Check sheet for the modelled part. Datum: model origin and axes. Units: mm. Face numbers are marked on the shaded views. Round coordinates to 2 decimals unless told otherwise and drop trailing zeros. Write each loop counter-clockwise with the first axis right and the second up, starting at its lowest first coordinate (ties: lowest second). Pieces come first, ordered by that corner, then holes. Notation, with made-up numbers: M 53.25,64.25 L 102.25,64.25 A15 cw 102.25,88.25 Z; hole C 72.5,70.25 d11. An arc over 180 degrees is marked long. Answer in a Markdown table with one row per item.
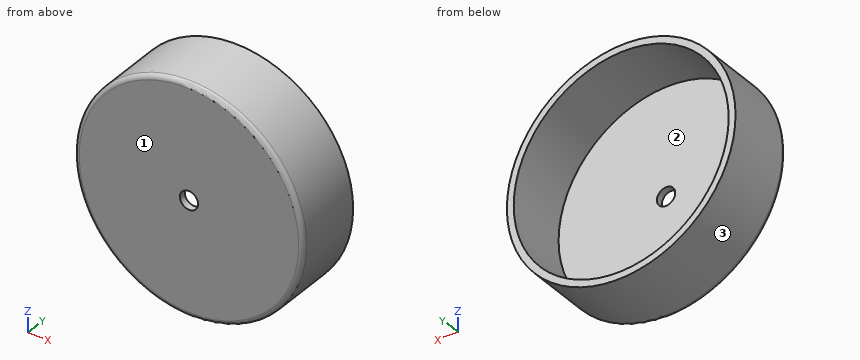
```python
from build123d import *

# Parameters (mm, degrees)
F0_R     = 50
F1_DEPTH = 30
F2_T     = -3
F3_R     = 2
F5_D     = 8


with BuildPart() as f1:
    # F0 (on Front) → F1 (new body)
    with BuildSketch(Plane.XZ):
        Circle(F0_R)
    extrude(amount=F1_DEPTH)

    # F2
    f2_openings = [f1.faces().sort_by_distance(p)[0] for p in [
        (0, 0, 0),
    ]]
    offset(amount=F2_T, openings=f2_openings)

    # F3
    f3_edges = [f1.edges().sort_by_distance(p)[0] for p in [
        (-50, -30, 0),
    ]]
    fillet(f3_edges, radius=F3_R)

    # F5 (through all)
    with Locations(Plane.XZ.offset(30)):
        with Locations((0, 0)):
            Hole(F5_D / 2)


solid = f1.part
```
1. Go/stop test with flat-tipped pins: pin 1 (1 mm diameter, centred on y = -6, z = 17, fed in from -X); pin 2 (3 mm diameter, centred on y = -4.5, z = 10.5, fed in from +X); pin 3 (1.5 mm diameter, centred on x = 38, y = -15.5, fed in from -Z); pin 4 (6.5 mm diameter, centred on x = 0, z = 0, fed in from +Y). Record where each tip stops, or that it passes through.
Found:
| item | result |
|---|---|
| pin 1 | stops at x = -47.2 |
| pin 2 | stops at x = 49.18 |
| pin 3 | stops at z = -33.35 |
| pin 4 | passes through |
2. Section check B-B, the plane z = 0. Record the cut outline in (x, y), and give its area (3 significant figures).
Found:
| item | result |
|---|---|
| outline | M -50,-28 A2 ccw -48,-30 L -4,-30 L -4,-27 L -47,-27 L -47,0 L -50,0 Z; M 4,-30 L 48,-30 A2 ccw 50,-28 L 50,0 L 47,0 L 47,-27 L 4,-27 Z |
| area | 436 mm2 |
3. Section check A-A, the plane x = 0. Record the cut outline in (y, z).
Found:
| item | result |
|---|---|
| outline | M -30,-48 A2 ccw -28,-50 L 0,-50 L 0,-47 L -27,-47 L -27,-4 L -30,-4 Z; M -30,4 L -27,4 L -27,47 L 0,47 L 0,50 L -28,50 A2 ccw -30,48 Z |
4. Draft check along Z on the marked faces 1, 2 and 3. Enter one of: +Z half, -Z half, draft (parallel to the pull), parting line (faces both ways), or undercut.
Found:
| item | result |
|---|---|
| face 1 | draft |
| face 2 | undercut |
| face 3 | parting line |
5. Section check C-C, the plane y = -10. Record the cut outline in (x, z), and give its area (3 significant figures).
Found:
| item | result |
|---|---|
| outline | C 0,0 d100; hole C 0,0 d94 |
| area | 914 mm2 |
6. Scan lines: L1, parallel to Z at x = 0, y = -6; L2, parallel to Y at x = -15, z = 19; L3, parallel to X at y = -8, z = -34.5. Record each from-to range of solid material in increasing order.
Found:
| item | result |
|---|---|
| L1 | z = -50 to -47, 47 to 50 |
| L2 | y = -30 to -27 |
| L3 | x = -36.19 to -31.92, 31.92 to 36.19 |
